```python
from build123d import *

# Parameters (mm, degrees)
ESBO_O1_W                = 34
ESBO_O1_H                = 35
ESBO_O1_R                = 1.5
ESBO_O1_W_2              = 23
ESBO_O1_H_2              = 6
RESSALTO_EXTRUS_O1_DEPTH = 2
ESBO_O2_W                = 34
ESBO_O2_H                = 2
RESSALTO_EXTRUS_O2_DEPTH = 15
ESBO_O3_R                = 1.75
CORTE_EXTRUS_O1_DEPTH    = 15


with BuildPart() as part:
    # Esboço1 → Ressalto-extrusão1 (new body)
    with BuildSketch(Plane.XY):
        with Locations((-5.310292873, -3.170678153)):
            Rectangle(ESBO_O1_W, ESBO_O1_H)
        with Locations((-19.810292873, 11.829321847)):
            Circle(ESBO_O1_R, mode=Mode.SUBTRACT)
        with Locations((9.189707127, 11.829321847)):
            Circle(ESBO_O1_R, mode=Mode.SUBTRACT)
        with Locations((-19.810292873, -18.170678153)):
            Circle(ESBO_O1_R, mode=Mode.SUBTRACT)
        with Locations((9.189707127, -18.170678153)):
            Circle(ESBO_O1_R, mode=Mode.SUBTRACT)
        with BuildLine():
            Line((-13.810292873, -1.170678153), (-13.810292873, -7.170678153))
            Line((-13.810292873, -7.170678153), (3.189707127, -7.170678153))
            Line((3.189707127, -7.170678153), (3.189707127, -1.170678153))
            Line((3.189707127, -1.170678153), (4.739707127, -1.170678153))
            ThreePointArc((4.739707127, -1.170678153), (6.472118741, -0.453089767), (7.189707127, 1.279321847))
            Line((7.189707127, 1.279321847), (7.189707127, 1.379321847))
            ThreePointArc((7.189707127, 1.379321847), (6.472118741, 3.11173346), (4.739707127, 3.829321847))
            Line((4.739707127, 3.829321847), (3.189707127, 3.829321847))
            Line((3.189707127, 3.829321847), (3.189707127, 11.829321847))
            Line((3.189707127, 11.829321847), (-13.810292873, 11.829321847))
            Line((-13.810292873, 11.829321847), (-13.810292873, 3.829321847))
            Line((-13.810292873, 3.829321847), (-15.360292873, 3.829321847))
            ThreePointArc((-15.360292873, 3.829321847), (-17.092704487, 3.11173346), (-17.810292873, 1.379321847))
            Line((-17.810292873, 1.379321847), (-17.810292873, 1.279321847))
            ThreePointArc((-17.810292873, 1.279321847), (-17.092704487, -0.453089767), (-15.360292873, -1.170678153))
            Line((-15.360292873, -1.170678153), (-13.810292873, -1.170678153))
        make_face(mode=Mode.SUBTRACT)
        with Locations((-5.310292873, -14.170678153)):
            Rectangle(ESBO_O1_W_2, ESBO_O1_H_2, mode=Mode.SUBTRACT)
    extrude(amount=RESSALTO_EXTRUS_O1_DEPTH)

    # Esboço2 → Ressalto-extrusão2 (add)
    with BuildSketch(Plane.XY.offset(2)):
        with Locations((-5.310292873, -21.670678153)):
            Rectangle(ESBO_O2_W, ESBO_O2_H)
    extrude(amount=-RESSALTO_EXTRUS_O2_DEPTH)

    # Esboço3 → Corte-extrusão1 (cut)
    with BuildSketch(Plane(origin=(0, -20.670678153, 0), x_dir=(1, 0, 0), z_dir=(0, 1, 0))):
        with Locations((8.189707127, 7.5)):
            Circle(ESBO_O3_R)
        with Locations((-18.810292873, 7.5)):
            Circle(ESBO_O3_R)
    extrude(amount=-CORTE_EXTRUS_O1_DEPTH, mode=Mode.SUBTRACT)


solid = part.part
```
The listing builds one solid part. Answer for the finished solid, in the listing's coordinates (mm). A direction names the side the tool comes from. Give positions to 0.01 mm unless a question says otherwise; leave off trailing zeros. Order: outer loops, then holes, each group sorted by start corner. A loop starts at its lowest first (then second) coordinate and runs counter-clockwise, first axis right, second up. Notation, with made-up numbers: (-29, 71) - (21, 71) arc R13 ccw to (21, 80) - close; hole circle Ø11 at (55, 80.5). An arc over 180 degrees is marked (long way). Use one line per item in the form item = value. Start each with the question number.
(1) A cutting plane is placed at B-B, the plane y = -3. Write down the section's boundary in (x, z).
(2) Flat-ended cylindrical pins translate along their axes: pin 1 Ø2 at (x, y) = (1, -16.5) entering from -Z; pin 2 Ø5 at (x, z) = (-17.5, -6.5) entering from +Y. Find the tip coordinate at first contact, or state that the pin passes through.
(3) The mould has two halves that part along Y. Classify faces 1 (the flat face through (-13.81, -4, 1)), 2 (the flat face through (-6, -20.671, -6)), 3 (the cylindrical face through (10, -16.91, 0.99)), 4 (the cylindrical face through (-17.194, -21.657, -6.83)): released by +Y, released by -Y, zero draft, split by the parting line, or undercut.
(4) For faces 5 (the cylindrical face through (6.44, -21.66, -7.58)), 6 (the flat face through (-15, -1.171, 1)), determine the directions among +Z, -Z, +X, -X, +Y, -Y from which every point of the face is accessible in a straight line to the end or side of a thin tool.
(5) A cutting plane is placed at C-C, the plane x = 1. Write down the section's boundary in (y, z), then the cut area to 3 significant figures.
(6) A cutting plane is placed at D-D, the plane x = 8.5. Write down the section's boundary in (y, z).
(7) Consider line 1 (Y direction, x = -7, z = 0.75); line 2 (X direction, y = -21.7, z = -7.5); line 3 (Z direction, x = -21, y = 5.5). Determine where each line is inside the solid, lowest interval first. Write a range as from..to.
(8) A cutting plane is placed at A-A, the plane z = -7.5. Write down the section's boundary in (x, y), then the cut area to 3 significant figures.
Ans:
q1.outline = (-22.31, 0) - (-13.81, 0) - (-13.81, 2) - (-22.31, 2) - close; (3.19, 0) - (11.69, 0) - (11.69, 2) - (3.19, 2) - close
q2.pin_1 = 0
q2.pin_2 = -20.67
q3.face_1 = undercut
q3.face_2 = released by +Y
q3.face_3 = undercut
q3.face_4 = zero draft
q4.face_5 = +Y, -Y
q4.face_6 = +Z, -Z
q5.outline = (-22.67, -13) - (-20.67, -13) - (-20.67, 0) - (-17.17, 0) - (-17.17, 2) - (-22.67, 2) - close; (-11.17, 0) - (-7.17, 0) - (-7.17, 2) - (-11.17, 2) - close; (11.83, 0) - (14.33, 0) - (14.33, 2) - (11.83, 2) - close
q5.area = 50.0 mm^2
q6.outline = (-22.67, -13) - (-20.67, -13) - (-20.67, -9.22) - (-22.67, -9.22) - close; (-22.67, -5.78) - (-20.67, -5.78) - (-20.67, 0) - (-19.5, 0) - (-19.5, 2) - (-22.67, 2) - close; (-16.84, 0) - (10.5, 0) - (10.5, 2) - (-16.84, 2) - close; (13.16, 0) - (14.33, 0) - (14.33, 2) - (13.16, 2) - close
q7.line_1 = -22.67..-17.17, -11.17..-7.17, 11.83..14.33
q7.line_2 = -22.31..-20.56, -17.06..6.44, 9.94..11.69
q7.line_3 = 0..2
q8.outline = (-22.31, -22.67) - (-20.56, -22.67) - (-20.56, -20.67) - (-22.31, -20.67) - close; (-17.06, -22.67) - (6.44, -22.67) - (6.44, -20.67) - (-17.06, -20.67) - close; (9.94, -22.67) - (11.69, -22.67) - (11.69, -20.67) - (9.94, -20.67) - close
q8.area = 54.0 mm^2
